from build123d import *

# Parameters (mm, degrees)
ESQUISSE1_W             = 19.5
ESQUISSE1_H             = 12.5
BOSS_EXTRU_1_DEPTH      = 0.8
ESQUISSE2_R             = 1.3
ENL_V_MAT_EXTRU_1_DEPTH = 0.8


with BuildPart() as part:
    # Esquisse1 → Boss.-Extru.1 (new body)
    with BuildSketch(Plane.XY):
        Rectangle(ESQUISSE1_W, ESQUISSE1_H)
    extrude(amount=BOSS_EXTRU_1_DEPTH)

    # Esquisse2 → Enlèv. mat.-Extru.1 (cut)
    with BuildSketch(Plane.XY.offset(0.8)):
        with Locations((-6.75, 3.25)):
            Circle(ESQUISSE2_R)
    extrude(amount=-ENL_V_MAT_EXTRU_1_DEPTH, mode=Mode.SUBTRACT)


solid = part.part
Verification items for the finished model (mm, model axes). Give positions to 0.01 mm unless a question says otherwise; leave off trailing zeros. Write each loop counter-clockwise with the first axis right and the second up, starting at its lowest first coordinate (ties: lowest second). Pieces come first, ordered by that corner, then holes. Notation, with made-up numbers: M 7,65 L 66,65 A36 ccw 66,100 Z; hole C 9.5,75 d3. An arc over 180 degrees is marked long. Use CSV: the item, a comma, the result in double quotes.
1) Cross-section at C-C (z = 0.4). Enter the section's corners in (x, y).
Final values:
outline,"M -9.75,-6.25 L 9.75,-6.25 L 9.75,6.25 L -9.75,6.25 Z; hole C -6.75,3.25 d2.6"
2) Material ranges on line 1 along Y through (x, z) = (-6.75, 0.5); line 2 along Y through (x, z) = (-7.25, 0.65), recorded low to high.
Final values:
line 1,"-6.25 to 1.95, 4.55 to 6.25"
line 2,"-6.25 to 2.05, 4.45 to 6.25"
3) Go/stop test with a flat-tipped pin: pin 1 Ø2 at (x, y) = (-6.75, 3.25) entering from -Z. Record where the tip stops, or that it passes through.
Final values:
pin 1,"through"
4) Cross-section at B-B (x = -6.75). Enter the section's corners in (y, z).
Final values:
outline,"M -6.25,0 L 1.95,0 L 1.95,0.8 L -6.25,0.8 Z; M 4.55,0 L 6.25,0 L 6.25,0.8 L 4.55,0.8 Z"
5) Cross-section at A-A (y = 3.25). Enter the section's corners in (x, z).
Final values:
outline,"M -9.75,0 L -8.05,0 L -8.05,0.8 L -9.75,0.8 Z; M -5.45,0 L 9.75,0 L 9.75,0.8 L -5.45,0.8 Z"
